Work out the finished part from the listing and answer in its coordinate system (mm). A direction names the side the tool comes from. Give positions to 0.01 mm unless a question says otherwise; leave off trailing zeros. Loops run counter-clockwise (first coordinate to the right, second up) from the corner with the lowest first, then second, coordinate; pieces in that order, holes last. Notation, with made-up numbers: (-0.5, 87.25) - (44.5, 87.25) arc R27 ccw to (44.5, 110.25) - close; hole circle Ø5 at (-31.75, -19.75). An arc over 180 degrees is marked (long way). Use one line per item in the form item = value. Start each with the question number.
Autodesk Inventor part; units mm, degrees
ref_plane "YZ Plane" through (0, 0, 0) normal (1, 0, 0) x (0, 1, 0)
ref_plane "XZ Plane" through (0, 0, 0) normal (0, 1, 0) x (-1, 0, 0)
ref_plane "XY Plane" through (0, 0, 0) normal (0, 0, 1) x (1, 0, 0)
sketch "Skizze1" plane through (0, 0, 0) normal (0, 0, 1) x (1, 0, 0)
  line L0 (0, 0) -> (0, 46.8858)
  line L1 (0, 46.8858) -> (-38, 15)
  line L2 (-38, 15) -> (-38, 0)
  line L3 (-38, 0) -> (0, 0)
  line L4 (-6.5, 6.5) -> (-6.5, 32.9465)
  line L5 (-6.5, 32.9465) -> (-31.5, 11.969)
  line L6 (-31.5, 11.969) -> (-31.5, 6.5)
  line L7 (-31.5, 6.5) -> (-6.5, 6.5)
  dimension "d0" = 130
  dimension "d1" = 15
  dimension "d2" = 38
  dimension "d3" = 6.5
  dimension "d4" = 6.5
  dimension "d6" = 6.5
  dimension "d7" = 6.5
extrude "Extrusion1" add sketch "Skizze1" along normal blind 12
sketch "Skizze2" plane through (0, 0, 12) normal (0, 0, 1) x (1, 0, 0)
  line L0 (-3, 40.4523) -> (-3, 3)
  line L1 (-3, 3) -> (-35, 3)
  line L2 (-35, 3) -> (-35, 13.6011)
  line L3 (-35, 13.6011) -> (-3, 40.4523)
  line L4 (-38, 0) -> (0, 0)
  line L5 (-38, 15) -> (-38, 0)
  line L6 (0, 46.8858) -> (-38, 15)
  line L7 (0, 0) -> (0, 46.8858)
  dimension "d10" = 3
  dimension "d11" = 3
  dimension "d12" = 3
  dimension "d13" = 3
extrude "Extrusion2" cut sketch "Skizze2" against normal blind 9 contours L0 L1 L2 L3
sketch "Skizze3" plane through (-35, 3, 12) normal (0, 1, 0) x (1, 0, 0)
  line L0 (35, 12) -> (35, 0)
  line L1 (35, 0) -> (32, 0)
  line L2 (32, 0) -> (32, 9)
  line L3 (32, 9) -> (0, 9)
  line L4 (0, 9) -> (0, 0)
  line L5 (0, 0) -> (-3, 0)
  line L6 (-3, 0) -> (-3, 12)
  line L7 (-3, 12) -> (35, 12)
  line L8 (32, 0) -> (0, 0)
  line L9 (0, 4.5) -> (32, 4.5)
  point P0 (6, 4.5)
  point P1 (26, 4.5)
  dimension "d17" = 6
  dimension "d18" = 6
hole "Bohrung1" at (-29, 3, 7.5) at (-9, 3, 7.5) direction (0, -1, 0) diameter 2.7 depth 8 tip angle 118
fillet "Rundung2" radius 1 9 edges at (0, 46.8858, 6) (-6.5, 32.9465, 1.5) (-3, 40.4523, 7.5) (-31.5, 6.5, 1.5) (-35, 3, 7.5) (-35, 13.6011, 7.5) (-31.5, 11.969, 1.5) (-3, 3, 7.5) (-6.5, 6.5, 1.5)
sketch "Skizze4" plane through (-34.6428, 13.9008, 3) normal (0.6427876, -0.7660444, 0) x (0.7660444, 0.6427876, 0)
  line L0 (45.2229, -3) -> (-4.3825, -3)
  line L1 (-4.3825, -3) -> (-4.3825, 9)
  line L2 (-4.3825, 9) -> (0, 9)
  line L3 (0, 0) -> (0, 9)
  line L4 (0, 0) -> (39.1622, 0)
  line L5 (39.1622, 0) -> (39.1622, 9)
  line L6 (0, 9) -> (39.1622, 9)
  line L7 (45.2229, 9) -> (45.2229, -3)
  line L8 (39.1622, 9) -> (45.2229, 9)
  point P0 (17.6026, -3)
  point P1 (4, 6.5)
  point P2 (35, 6.5)
  dimension "d27" = 2.5
  dimension "d28" = 4
  dimension "d29" = 2.5
  dimension "d30" = 35
  dimension "d31" = 4.1622
hole "Bohrung2" at (-31.5786, 16.472, 9.5) at (-7.8312, 36.3984, 9.5) direction (-0.6427876, 0.7660444, 0) diameter 2.7 depth 8 tip angle 118
sketch "Skizze7" plane through (-38, 15, 12) normal (-0.6427876, 0.7660444, 0) x (0.7660444, 0.6427876, 0)
  circle A0 centre (36.8652, 2.5) radius 1.35
  line L0 (38.2152, 2.5) -> (38.2152, 0)
  line L1 (1.8652, 0) -> (41.0274, 0)
  line L2 (35.5152, 0) -> (35.5152, 2.5)
  point P0 (19.4679, 12)
extrude "Extrusion3" cut sketch "Skizze7" against normal blind 6.25 contours L0 L1 L2 A0
sketch "Skizze8" plane through (-38, 15, 12) normal (-0.6427876, 0.7660444, 0) x (0.7660444, 0.6427876, 0)
  circle A0 centre (5.8652, 2.5) radius 1.35
  line L0 (7.2152, 2.5) -> (7.2152, 0)
  line L1 (-9.6418, 0) -> (19.4679, 0)
  line L2 (4.5152, 2.5) -> (4.5152, 0)
  point P0 (19.4679, 12)
extrude "Extrusion4" cut sketch "Skizze8" against normal blind 6.5 contours L0 L1 L2 A0
properties part number "lcd_halterung_162C_rechts"
1) Flat-ended cylindrical pins translate along their axes: pin 1 Ø4 at (y, z) = (28.5, 5.5) entering from -X; pin 2 Ø1 at (x, z) = (-15.5, 4.5) entering from +Y; pin 3 Ø7 at (y, z) = (22.5, 9.5) entering from -X. Find the tip coordinate at first contact, or state that the pin passes through.
2) A cutting plane is placed at C-C (y = 3.5). Give the vertices of the cut face in (x, z), plus the area to 3 significant figures.
3) Find the intervals of material crossed by probe 1 along X at (y, z) = (2.25, 7.5); probe 2 along Z at (x, y) = (-9, 2.45); probe 3 along Z at (x, y) = (-3.5, 4), in increasing order.
4) Determine the mould class of faces 1 (the cylindrical face through (-3.59, 39.22, 7.44)), 2 (the flat face through (-33.59, 16.77, 10.73)), 3 (the flat face through (-19, 23, 0)), 4 (the cylindrical face through (-8.79, 37.58, 8.15)) for opening direction Y: released by +Y, released by -Y, zero draft, split by the parting line, or undercut.
5) A cutting plane is placed at D-D (x = -29). Give the vertices of the cut face in (y, z).
6) A cutting plane is placed at A-A (z = 7.5). Give the vertices of the cut face in (x, y), plus the area to 3 significant figures.
7) A cutting plane is placed at B-B (x = -21). Give the vertices of the cut face in (y, z), plus the area to 3 significant figures.
8) A tool of negligible diameter and unlimited length cuts with its end or side. For faces 5 (the flat face through (-31.52, 18.5, 10.73)), 6 (the flat face through (-9.843, 36.696, 10.768)), 7 (the cylindrical face through (-6.801, 6.785, 1.521)), 8 (the cylindrical face through (-27.8, 1.48, 8.12)), from which of +Z, -Z, +X, -X, +Y, -Y can it reach the whole face along a straight path? Write none if from no direction.
Answer sheet:
q1.pin_1 = -24.29
q1.pin_2 = 34.3
q1.pin_3 = -32.99
q2.outline = (-38, 0) - (0, 0) - (0, 12) - (-3.13, 12) - (-3.13, 3) - (-34.87, 3) - (-34.87, 12) - (-38, 12) - close
q2.area = 170 mm²
q3.probe_1 = -38 to -30.35, -27.65 to -10.35, -7.65 to 0
q3.probe_2 = 0 to 6.15, 8.85 to 12
q3.probe_3 = 0 to 3
q4.face_1 = undercut
q4.face_2 = released by +Y
q4.face_3 = zero draft
q4.face_4 = undercut
q5.outline = (0, 0) - (6.5, 0) - (6.5, 3) - (3, 3) - (3, 6.15) - (0, 6.15) - close; (0, 8.85) - (3, 8.85) - (3, 12) - (0, 12) - close; (14.07, 0) - (22.55, 0) - (22.55, 12) - (18.64, 12) - (18.64, 3) - (14.07, 3) - close
q6.outline = (-38, 0) - (-30.35, 0) - (-30.35, 3) - (-34, 3) arc R1 cw to (-35, 4) - (-35, 13.13) arc R1 cw to (-34.64, 13.9) - (-4.64, 39.07) arc R1 cw to (-3, 38.31) - (-3, 4) arc R1 cw to (-4, 3) - (-7.65, 3) - (-7.65, 0) - (0, 0) - (0, 44.74) arc R1 ccw to (-1.64, 45.51) - (-38, 15) - close; (-27.65, 0) - (-10.35, 0) - (-10.35, 3) - (-27.65, 3) - close
q6.area = 391 mm²
q7.outline = (0, 0) - (6.5, 0) - (6.5, 3) - (3, 3) - (3, 12) - (0, 12) - close; (20.78, 0) - (29.26, 0) - (29.26, 12) - (25.35, 12) - (25.35, 3) - (20.78, 3) - close
q7.area = 107 mm²
q8.face_5 = +Z
q8.face_6 = +Z, +Y
q8.face_7 = +Z, -Z
q8.face_8 = -Y
